Check sheet for the modelled part. Datum: model origin and axes. Units: mm. A direction names the side the tool comes from. Round coordinates to 2 decimals unless told otherwise and drop trailing zeros. Write each loop counter-clockwise with the first axis right and the second up, starting at its lowest first coordinate (ties: lowest second). Pieces come first, ordered by that corner, then holes.
Autodesk Inventor part; units mm, degrees
ref_plane "YZ Plane" through (0, 0, 0) normal (1, 0, 0) x (0, 1, 0)
ref_plane "XZ Plane" through (0, 0, 0) normal (0, 1, 0) x (-1, 0, 0)
ref_plane "XY Plane" through (0, 0, 0) normal (0, 0, 1) x (1, 0, 0)
sketch "Sketch1" plane through (0, 0, 0) normal (0, 0, 1) x (1, 0, 0)
  line L0 (0, 0) -> (-50, 0)
  line L1 (-50, 0) -> (-50, 30)
  line L2 (-50, 30) -> (0, 30)
  line L3 (0, 30) -> (0, 0)
  line L4 (-50, 30) -> (-80, 30)
  line L5 (-80, 30) -> (-80, -20)
  line L6 (-80, -20) -> (-50, -20)
  line L7 (-50, -20) -> (-50, 30)
  line L8 (-80, 0) -> (-50, 0)
  dimension "d0" = 50
  dimension "d1" = 30
  dimension "d2" = 30
  dimension "d3" = 50
extrude "Extrusion1" add sketch "Sketch1" along normal blind 30
fillet "Fillet1" radius 2 12 edges at (-40, 30, 30) (0, 15, 30) (-25, 0, 30) (-50, -10, 30) (-50, -20, 15) (-65, -20, 30) (0, 30, 15) (0, 0, 15) (-40, 30, 0) (-80, 30, 15) (-80, 5, 30) (-80, 5, 0)
properties part number "elbow"
1. Sectioned sample at C-C, the plane x = -10. Enter the section's corners in (y, z).
2. Sectioned sample at A-A, the plane y = -2. Enter the section's corners in (x, z).
3. Sectioned sample at B-B, the plane z = 15. Enter the section's corners in (x, y).
4. Set-up check for faces 1 (the flat face through (-66, -20, 14)), 2 (the flat face through (-50, -9, 14)), 3 (the cylindrical face through (-50.6, -7.86, 29.43)): record each of +Z, -Z, +X, -X, +Y, -Y from which the full face is reachable in a straight line by a thin tool's end or side.
5. Scan lines: line 1 along Y through (x, z) = (-38, 19.5); line 2 along X through (y, z) = (-8.5, 12.5); line 3 along X through (y, z) = (0.5, 24). Record each from-to range of solid material in increasing order.
6. Go/stop test with flat-tipped pins: pin 1 (1 mm diameter, centred on y = 0, z = 17.5, fed in from +X); pin 2 (8.5 mm diameter, centred on x = -33, z = 7, fed in from -Y); pin 3 (5.5 mm diameter, centred on y = -8.5, z = 11.5, fed in from +X). Record where each tip stops, or that it passes through.
Computed values:
1. outline: (0, 0) - (28, 0) arc R2 ccw to (30, 2) - (30, 28) arc R2 ccw to (28, 30) - (2, 30) arc R2 ccw to (0, 28) - close
2. outline: (-80, 2) arc R2 ccw to (-78, 0) - (-50, 0) - (-50, 28) arc R2 ccw to (-52, 30) - (-78, 30) arc R2 ccw to (-80, 28) - close
3. outline: (-80, -20) - (-52, -20) arc R2 ccw to (-50, -18) - (-50, 0) - (-2, 0) arc R2 ccw to (0, 2) - (0, 28) arc R2 ccw to (-2, 30) - (-78, 30) arc R2 ccw to (-80, 28) - close
4. face 1: +Z, -Z, +X, -X, -Y
4. face 2: +Z, -Z, +X, -Y
4. face 3: +Z, +X, -Y
5. line 1: y = 0 to 30
5. line 2: x = -80 to -50
5. line 3: x = -80 to -0.68
6. pin 1: stops at x = -0.68
6. pin 2: stops at y = 0
6. pin 3: stops at x = -50
